Work out the finished part from the listing and answer in its coordinate system (mm). A direction names the side the tool comes from. Coordinates: 2 decimals unless noted, no trailing zeros. Loops run counter-clockwise (first coordinate to the right, second up) from the corner with the lowest first, then second, coordinate; pieces in that order, holes last. Notation, with made-up numbers: (86, 23.25) -> (120, 23.25) arc R12 ccw to (120, 43.25) -> close; hole circle Ø3 at (59, 11). An arc over 180 degrees is marked (long way). Use a Markdown table: item, result.
from build123d import *

# Parameters (mm, degrees)
F0_W     = 57.15
F0_H     = 101.6
F1_DEPTH = 6.35
F3_DEPTH = 76.2
F4_R     = 12.7
F5_DEPTH = 6.35
F7_R     = 12.7
F8_DEPTH = 6.35


with BuildPart() as f1:
    # F0 (on Top) → F1 (new body)
    with BuildSketch(Plane.XY):
        with Locations((-28.575, 0)):
            Rectangle(F0_W, F0_H)
    extrude(amount=F1_DEPTH)

    # F2 (on face) → F3 (join)
    with BuildSketch(Plane.XY.offset(6.35)):
        Polygon((-50.8, 50.8), (-57.15, 50.8), (-57.15, -44.45), (-133.35, -44.45), (-133.35, -50.8), (0, -50.8), (0, -44.45), (-50.8, -44.45), align=None)
    extrude(amount=F3_DEPTH)

    # F4 (on face) → F5 (cut, through all)
    with BuildSketch(Plane(origin=(-57.15, 0, 0), x_dir=(0, -1, 0), z_dir=(-1, 0, 0))):
        with Locations((0, 57.15)):
            Circle(F4_R)
    extrude(amount=-F5_DEPTH, mode=Mode.SUBTRACT)

    # F6: F1 across plane


with BuildPart() as f1_1:
    add(f1.part)
    add(f1.part.mirror(Plane.YZ))

    # F7 (on face) → F8 (cut, through all)
    with BuildSketch(Plane(origin=(0, -44.45, 0), x_dir=(-1, 0, 0), z_dir=(0, 1, 0))):
        with Locations((0, 38.1)):
            Circle(F7_R)
    extrude(amount=-F8_DEPTH, mode=Mode.SUBTRACT)


solid = f1_1.part
Q1. Consider line 1 (X direction, y = 17, z = 70); line 2 (Z direction, x = -53, y = 0); line 3 (Z direction, x = 0, y = -47.5). Determine where each line is inside the solid, lowest interval first. Write a range as [from, to].
Solved:
| item | result |
|---|---|
| line 1 | [-57.15, -50.8], [50.8, 57.15] |
| line 2 | [0, 44.45], [69.85, 82.55] |
| line 3 | [0, 25.4], [50.8, 82.55] |
Q2. Section A-A on y = 0 is taken. Determine the outline of the cut face in (x, z).
Solved:
| item | result |
|---|---|
| outline | (-57.15, 0) -> (57.15, 0) -> (57.15, 44.45) -> (50.8, 44.45) -> (50.8, 6.35) -> (-50.8, 6.35) -> (-50.8, 44.45) -> (-57.15, 44.45) -> close; (-57.15, 69.85) -> (-50.8, 69.85) -> (-50.8, 82.55) -> (-57.15, 82.55) -> close; (50.8, 69.85) -> (57.15, 69.85) -> (57.15, 82.55) -> (50.8, 82.55) -> close |
Q3. Section B-B on x = 0 is taken. Determine the outline of the cut face in (y, z).
Solved:
| item | result |
|---|---|
| outline | (-50.8, 0) -> (50.8, 0) -> (50.8, 6.35) -> (-44.45, 6.35) -> (-44.45, 25.4) -> (-50.8, 25.4) -> close; (-50.8, 50.8) -> (-44.45, 50.8) -> (-44.45, 82.55) -> (-50.8, 82.55) -> close |
Q4. Determine the mould class of faces 1 (the flat face through (-96, -48, 6.35)), 2 (the cylindrical face through (54.02, 2.75, 44.75)), 3 (the flat face through (-1, -44.45, 52)) for opening direction Y: pulls with the +Y half, pulls with the -Y half, needs draft (parallel to the pull), parting line crosses it, or undercut.
Solved:
| item | result |
|---|---|
| face 1 | needs draft |
| face 2 | undercut |
| face 3 | pulls with the +Y half |
Q5. Given pin 1 Ø8 at (y, z) = (-28.5, 53) entering from -X; pin 2 Ø3 at (y, z) = (-14, 23.5) entering from +X; pin 3 Ø3 at (x, z) = (-6.5, 74) entering from +Y; pin 4 Ø20.5 at (y, z) = (0, 57.15) entering from -X, each flat-ended and moving along its own axis, determine where each tip first touches the part or whether it passes through.
Solved:
| item | result |
|---|---|
| pin 1 | x = -57.15 |
| pin 2 | x = 57.15 |
| pin 3 | y = -44.45 |
| pin 4 | through |
Q6. Section C-C on z = 38.1 is taken. Determine the outline of the cut face in (x, y), and give its area (3 significant figures).
Solved:
| item | result |
|---|---|
| outline | (-133.35, -50.8) -> (-12.7, -50.8) -> (-12.7, -44.45) -> (-50.8, -44.45) -> (-50.8, 50.8) -> (-57.15, 50.8) -> (-57.15, -44.45) -> (-133.35, -44.45) -> close; (12.7, -50.8) -> (133.35, -50.8) -> (133.35, -44.45) -> (57.15, -44.45) -> (57.15, 50.8) -> (50.8, 50.8) -> (50.8, -44.45) -> (12.7, -44.45) -> close |
| area | 2,740 mm² |
Q7. Section D-D on y = 41 is taken. Determine the outline of the cut face in (x, z).
Solved:
| item | result |
|---|---|
| outline | (-57.15, 0) -> (57.15, 0) -> (57.15, 82.55) -> (50.8, 82.55) -> (50.8, 6.35) -> (-50.8, 6.35) -> (-50.8, 82.55) -> (-57.15, 82.55) -> close |
Q8. For faces 4 (the flat face through (96, -48, 6.35)), 5 (the flat face through (-95, -44.45, 44)), 6 (the flat face through (50.8, 3, 44)), determine the directions among +Z, -Z, +X, -X, +Y, -Y from which every point of the face is accessible in a straight line to the end or side of a thin tool.
Solved:
| item | result |
|---|---|
| face 4 | -Z, +X, +Y, -Y |
| face 5 | +Z, -Z, -X, +Y |
| face 6 | +Z, +Y |
